Design review of the part built by this model. Coordinates are the model's own, in mm. A direction names the side the tool comes from. Give positions to 0.01 mm unless a question says otherwise; leave off trailing zeros. Order: outer loops, then holes, each group sorted by start corner. A loop starts at its lowest first (then second) coordinate and runs counter-clockwise, first axis right, second up. Notation, with made-up numbers: (10, 19) -> (61, 19) arc R25 ccw to (61, 57) -> close; hole circle Ø4 at (62, 79.5). An arc over 180 degrees is marked (long way). Return JSON: item names as keys, results as strings.
```python
from build123d import *

# Parameters (mm, degrees)
CROQUIS1_W                   = 270
CROQUIS1_H                   = 240
SALIENTE_EXTRUIR1_DEPTH      = 30
CROQUIS1_W_2                 = 116.5
SALIENTE_EXTRUIR1_2_DEPTH    = 30
SALIENTE_EXTRUIR3_DEPTH      = 63.5
CROQUIS3_W                   = 406.759820342
CROQUIS3_H                   = 44.054315541
SALIENTE_EXTRUIR4_DEPTH      = 245.5
CROQUIS4_R                   = 38.153863336
CROQUIS4_R_2                 = 29.41561916
SALIENTE_EXTRUIR5_DEPTH      = 3
CROQUIS5_R                   = 4.7645
CORTAR_EXTRUIR1_DEPTH        = 142
CROQUIS6_W                   = 6.655343447
CROQUIS6_H                   = 44.054315541
SALIENTE_EXTRUIR6_DEPTH      = 294
SALIENTE_EXTRUIR6_DEPTH_BACK = 113
CROQUIS7_R                   = 1.651
SALIENTE_EXTRUIR8_DEPTH      = 112
SALIENTE_EXTRUIR8_DEPTH_BACK = 2
CROQUIS8_W                   = 3.302
CROQUIS8_H                   = 24.988896413
CORTAR_EXTRUIR2_DEPTH        = 112


with BuildPart() as part:
    # Croquis1 → Saliente-Extruir1 (new body)
    with BuildSketch(Plane(origin=(0, 0, 0), x_dir=(1, 0, 0), z_dir=(0, 1, 0))):
        with Locations((32.193078438, 120)):
            Rectangle(CROQUIS1_W, CROQUIS1_H)
    extrude(amount=SALIENTE_EXTRUIR1_DEPTH)



with BuildPart() as body_2:
    # Croquis1 → Saliente-Extruir1 2 (new body)
    with BuildSketch(Plane(origin=(0, 0, 0), x_dir=(1, 0, 0), z_dir=(0, 1, 0))):
        with Locations((229.288362697, 120)):
            Rectangle(CROQUIS1_W_2, CROQUIS1_H)
    extrude(amount=SALIENTE_EXTRUIR1_2_DEPTH)


with BuildPart() as part_1:
    add(part.part)

    add(body_2.part)  # Saliente-Extruir3 merges body 2
    # Croquis2 → Saliente-Extruir3 (add)
    with BuildSketch(Plane(origin=(0, 0, 0), x_dir=(1, 0, 0), z_dir=(0, 1, 0))):
        Polygon((-102.861944812, 0), (287.538362697, 0), (287.538362697, 240), (-102.806921562, 240), align=None)
    extrude(amount=-SALIENTE_EXTRUIR3_DEPTH)

    # Croquis3 → Saliente-Extruir4 (add)
    with BuildSketch(Plane.XY):
        with Locations((91.027758877, 22.027157771)):
            Rectangle(CROQUIS3_W, CROQUIS3_H)
    extrude(amount=-SALIENTE_EXTRUIR4_DEPTH)

    # Croquis4 → Saliente-Extruir5 (add)
    with BuildSketch(Plane(origin=(0, 44.054315541, 0), x_dir=(1, 0, 0), z_dir=(0, 1, 0))):
        with Locations((17.647848706, 101.450529821)):
            Circle(CROQUIS4_R)
        with Locations((17.647848706, 101.450529821)):
            Circle(CROQUIS4_R_2, mode=Mode.SUBTRACT)
    extrude(amount=SALIENTE_EXTRUIR5_DEPTH)

    # Croquis5 → Cortar-Extruir1 (cut)
    with BuildSketch(Plane(origin=(0, 0, 0), x_dir=(1, 0, 0), z_dir=(0, 1, 0))):
        with Locations((17.647848706, 101.450529821)):
            Circle(CROQUIS5_R)
    extrude(amount=CORTAR_EXTRUIR1_DEPTH, mode=Mode.SUBTRACT)

    # Croquis6 → Saliente-Extruir6 (add, two sides)
    with BuildSketch(Plane(origin=(0, 0, 0), x_dir=(0, 0, -1), z_dir=(1, 0, 0))) as saliente_extruir6_sk:
        with Locations((-3.327671724, 22.027157771)):
            Rectangle(CROQUIS6_W, CROQUIS6_H)
    extrude(amount=SALIENTE_EXTRUIR6_DEPTH)
    extrude(saliente_extruir6_sk.sketch, amount=-SALIENTE_EXTRUIR6_DEPTH_BACK)

    # Croquis7 → Saliente-Extruir8 (add, two sides)
    with BuildSketch(Plane(origin=(0, 0, 0), x_dir=(1, 0, 0), z_dir=(0, 1, 0))) as saliente_extruir8_sk:
        with Locations((269.705344772, 51.231276753)):
            Circle(CROQUIS7_R)
    extrude(amount=SALIENTE_EXTRUIR8_DEPTH)
    extrude(saliente_extruir8_sk.sketch, amount=-SALIENTE_EXTRUIR8_DEPTH_BACK)

    # Croquis8 → Cortar-Extruir2 (cut)
    with BuildSketch(Plane.XY):
        with Locations((269.705344772, 99.505551794)):
            Rectangle(CROQUIS8_W, CROQUIS8_H)
    extrude(amount=-CORTAR_EXTRUIR2_DEPTH, mode=Mode.SUBTRACT)


solid = part_1.part
```
Item 1: Machinability: for faces 1 (the face through (-112.352, 22, -121)), 2 (the face through (90, -31, 0)), 3 (the face through (287.538, -31, -118)), 4 (the face through (95, -31, -240)), 5 (the face through (14.136, 21.719, -104.671)), which of the approach directions +Z, -Z, +X, -X, +Y, -Y give a long, thin tool a straight path to every point of the face, cutting with its end or side? Answer none if there is none.
Result set:
{"face 1": "-Z, -X, +Y, -Y", "face 2": "+Z, +X, -X, -Y", "face 3": "+Z, -Z, +X, -Y", "face 4": "-Z, +X, -X, -Y", "face 5": "+Y"}
Item 2: Add section A-A (x = 234). Give the boundary of the cut face in (y, z), plus the area to 3 significant figures.
Result set:
{"outline": "(-63.5, -240) -> (0, -240) -> (0, -245.5) -> (44.05, -245.5) -> (44.05, 6.66) -> (0, 6.66) -> (0, 0) -> (-63.5, 0) -> close", "area": "26,300 mm^2"}
Item 3: Add section B-B (z = -161). Give the boundary of the cut face in (x, y).
Result set:
{"outline": "(-112.35, 0) -> (-102.83, 0) -> (-102.83, -63.5) -> (287.54, -63.5) -> (287.54, 0) -> (294.41, 0) -> (294.41, 44.05) -> (-112.35, 44.05) -> close"}
Item 4: Mouldability with a two-part tool opening along Z and no side actions: class faces 6 (the face through (88, 22, -245.5)), 7 (the face through (17, 44.054, -108)), 8 (the face through (93, 22, 6.655)), 9 (the face through (294.408, 22, -121)) as released by +Z, released by -Z, zero draft, split by the parting line, or undercut.
Result set:
{"face 6": "released by -Z", "face 7": "undercut", "face 8": "released by +Z", "face 9": "zero draft"}
Item 5: For pin 1 (5 mm diameter, centred on x = 18, z = -103, fed in from +Y); pin 2 (7.5 mm diameter, centred on y = 11.5, z = 4, fed in from +X); pin 3 (19 mm diameter, centred on x = 38, y = -31.5, fed in from -Z); pin 4 (0.7 mm diameter, centred on x = -112.5, y = 21, fed in from -Z), all flat-tipped, find the tip position at first contact; note any pin that passes through.
Result set:
{"pin 1": "stops at y = 0", "pin 2": "stops at x = 294", "pin 3": "stops at z = -240", "pin 4": "stops at z = -245.5"}
Item 6: Wall thickness on L1, parallel to X at y = -8.5, z = -220; L2, parallel to Z at x = 43, y = -42.5; L3, parallel to Y at x = 67.5, z = -190: over which ranges is each line inside the solid? List them lowest first. Write a range as [from, to].
Result set:
{"L1": "x = [-102.81, 287.54]", "L2": "z = [-240, 0]", "L3": "y = [-63.5, 44.05]"}
Item 7: Add section D-D (z = -89). Give the boundary of the cut face in (x, y).
Result set:
{"outline": "(-112.35, 0) -> (-102.84, 0) -> (-102.84, -63.5) -> (287.54, -63.5) -> (287.54, 0) -> (294.41, 0) -> (294.41, 44.05) -> (53.71, 44.05) -> (53.71, 47.05) -> (44.3, 47.05) -> (44.3, 44.05) -> (-9, 44.05) -> (-9, 47.05) -> (-18.42, 47.05) -> (-18.42, 44.05) -> (-112.35, 44.05) -> close"}
Item 8: Add section C-C (y = -27). Give the boundary of the cut face in (x, z).
Result set:
{"outline": "(-102.86, 0) -> (-102.81, -240) -> (287.54, -240) -> (287.54, 0) -> close"}
